Could you check a few things on this model? Use its own coordinates, in mm. A direction names the side the tool comes from. Round coordinates to 2 decimals unless told otherwise and drop trailing zeros. Loops run counter-clockwise (first coordinate to the right, second up) from the corner with the lowest first, then second, coordinate; pieces in that order, holes last. Notation, with made-up numbers: (-14.75, 37.25) -> (16.25, 37.25) arc R27 cw to (16.25, 70.25) -> close; hole circle Ø7 at (50, -20). An arc over 180 degrees is marked (long way). Use CSV: the item, a comma, the result in double quotes. Start each with the question number.
```python
from build123d import *


with BuildPart() as part:
    # Esquisse1 → Révolution1 (revolve)
    with BuildSketch(Plane.XY, mode=Mode.PRIVATE) as r_volution1_sk:
        Polygon((-2, 3.845299462), (-2, 0), (-3, 0), (-3, 3), (-10.5, 3), (-10.5, 4.5), (-6, 4.5), (-6, 12.5), (-4.5, 12.5), (-4.5, 9), (-4, 9), (-4, 5), align=None)
    revolve(r_volution1_sk.sketch.rotate(Axis((0, 0, 0), (0, 1, 0)), 270), axis=Axis((0, 0, 0), (0, 1, 0)))  # turned: the seam where the file's is


solid = part.part
```
1. Suppose I cut it at B-B (x = 0). List the corners of the cut face in (y, z) for me, then the cut area to 3 significant figures.
2. Will these pins go through, and if not, where does the flat tip stop? pin 1 (2 mm diameter, centred on y = 5, z = 4, fed in from +X); pin 2 (5 mm diameter, centred on x = -1, y = 8, fed in from -Z); pin 3 (6 mm diameter, centred on x = -5.5, z = 4, fed in from -Y).
3. Suppose I cut it at A-A (z = 0). List the corners of the cut face in (x, y) for me.
4. We'd pull the mould along Z, two halves only. Please class faces 1 (the face through (3, 9, 3)), 2 (the face through (-3.2, 3.8, -10)), 3 (the face through (-2.5, 3, 2.2)): pulls with the +Z half, pulls with the -Z half, needs draft (parallel to the pull), parting line crosses it, or undercut.
5. If I drill on L1, parallel to X at y = 7.15, z = 0; L2, parallel to X at y = 1.9, z = 0; L3, parallel to Y at x = 2.75, z = 8, over which ranges is the centre line in solid material (lowest first)?
6. Suppose I cut it at D-D (y = 11.75). List the corners of the cut face in (x, z) for me.
7. Suppose I cut it at C-C (y = 5.75). List the corners of the cut face in (x, z) for me.
8. For faces 4 (the face through (-1.352, 10.726, -4.292)), 5 (the face through (-0.9, 1.52, -2.86)), 6 (the face through (-4.5, 12.5, 1.4)), which set-ups out of +Z, -Z, +X, -X, +Y, -Y let a thin tool reach every point of the face, with its end or its side?
Geometry check:
1,outline,"(0, -3) -> (3, -3) -> (3, -10.5) -> (4.5, -10.5) -> (4.5, -6) -> (12.5, -6) -> (12.5, -4.5) -> (9, -4.5) -> (9, -4) -> (5, -4) -> (3.85, -2) -> (0, -2) -> close; (0, 2) -> (3.85, 2) -> (5, 4) -> (9, 4) -> (9, 4.5) -> (12.5, 4.5) -> (12.5, 6) -> (4.5, 6) -> (4.5, 10.5) -> (3, 10.5) -> (3, 3) -> (0, 3) -> close"
1,area,"59.7 mm²"
2,pin 1,"stops at x = 10.02"
2,pin 2,"stops at z = -6"
2,pin 3,"stops at y = 3"
3,outline,"(-10.5, 3) -> (-3, 3) -> (-3, 0) -> (-2, 0) -> (-2, 3.85) -> (-4, 5) -> (-4, 9) -> (-4.5, 9) -> (-4.5, 12.5) -> (-6, 12.5) -> (-6, 4.5) -> (-10.5, 4.5) -> close; (2, 0) -> (3, 0) -> (3, 3) -> (10.5, 3) -> (10.5, 4.5) -> (6, 4.5) -> (6, 12.5) -> (4.5, 12.5) -> (4.5, 9) -> (4, 9) -> (4, 5) -> (2, 3.85) -> close"
4,face 1,"undercut"
4,face 2,"parting line crosses it"
4,face 3,"needs draft"
5,L1,"x = -6 to -4, 4 to 6"
5,L2,"x = -3 to -2, 2 to 3"
5,L3,"y = 3 to 4.5"
6,outline,"circle Ø12 at (0, 0); hole circle Ø9 at (0, 0)"
7,outline,"circle Ø12 at (0, 0); hole circle Ø8 at (0, 0)"
8,face 4,"+Y"
8,face 5,"-Y"
8,face 6,"+Z, -Z, +X, -X, +Y"
